Geometry check sheet. Reference: the model listing, model coordinates, mm. Give positions to 0.01 mm unless a question says otherwise; leave off trailing zeros. Write each loop counter-clockwise with the first axis right and the second up, starting at its lowest first coordinate (ties: lowest second). Pieces come first, ordered by that corner, then holes. Notation, with made-up numbers: (71.5, 60.25) - (112.5, 60.25) arc R31 cw to (112.5, 89.25) - close; hole circle Ø4 at (36.25, 39). An arc over 180 degrees is marked (long way). Write item = value, one per line. Start each with the question number.
(1) Section check D-D, the plane y = 29. Enter the section's corners in (x, z), plus the area to 3 significant figures.
(2) Draft check along Y on faces 1 (the cylindrical face through (96, 34, 1)), 2 (the flat face through (109, 50, 2)). Enter one of: pulls with the +Y half, pulls with the -Y half, needs draft (parallel to the pull), parting line crosses it, or undercut.
(3) Depth check by flat-ended pin: pin 1 Ø2.5 at (x, y) = (2.5, 2.5) entering from -Z. Enter the tip coordinate at first touch or a pass-through.
(4) Section check C-C, the plane y = 72. Enter the section's corners in (x, z), plus the area to 3 significant figures.
(5) Thickness scan on L1, parallel to X at y = 95.5, z = 1.4; L2, parallel to Y at x = 2.5, z = 0.65; L3, parallel to Y at x = 94, z = 0.8. Record the ranges inside material, lowest first.
(6) Section check B-B, the plane z = 1.25. Give the number of separate pieces and of enclosed holes in the cut face, plus the area to 3 significant figures.
(7) Section check A-A, the plane x = 60. Enter the section's corners in (y, z), plus the area to 3 significant figures.
```python
from build123d import *

# Parameters (mm, degrees)
SKETCH_1_W      = 180
SKETCH_1_H      = 98
SKETCH_1_R      = 1.5
SKETCH_1_R_2    = 39
SKETCH_1_R_3    = 2
SKETCH_1_R_4    = 1.6
SKETCH_1_W_2    = 27.4
SKETCH_1_H_2    = 47.2
EXTRUDE_1_DEPTH = 2
FILLET_1_R      = 1
FILLET_2_R      = 1


with BuildPart() as part:
    # Эскиз1 → Бобышка-Вытянуть1 (new body)
    with BuildSketch(Plane.XY):
        with Locations((90, 49)):
            Rectangle(SKETCH_1_W, SKETCH_1_H)
        with Locations((2.5, 95.5)):
            Circle(SKETCH_1_R, mode=Mode.SUBTRACT)
        with Locations((177.5, 95.5)):
            Circle(SKETCH_1_R, mode=Mode.SUBTRACT)
        with Locations((177.5, 2.5)):
            Circle(SKETCH_1_R, mode=Mode.SUBTRACT)
        with Locations((2.5, 2.5)):
            Circle(SKETCH_1_R, mode=Mode.SUBTRACT)
        with Locations((60, 49)):
            Circle(SKETCH_1_R_2, mode=Mode.SUBTRACT)
        with Locations((24.25, 84.75)):
            Circle(SKETCH_1_R_3, mode=Mode.SUBTRACT)
        with Locations((95.75, 84.75)):
            Circle(SKETCH_1_R_3, mode=Mode.SUBTRACT)
        with Locations((95.75, 13.25)):
            Circle(SKETCH_1_R_3, mode=Mode.SUBTRACT)
        with Locations((24.25, 13.25)):
            Circle(SKETCH_1_R_3, mode=Mode.SUBTRACT)
        with Locations((125, 64.4)):
            Circle(SKETCH_1_R_4, mode=Mode.SUBTRACT)
        with Locations((165, 64.4)):
            Circle(SKETCH_1_R_4, mode=Mode.SUBTRACT)
        with Locations((145, 64.4)):
            Rectangle(SKETCH_1_W_2, SKETCH_1_H_2, mode=Mode.SUBTRACT)
    extrude(amount=EXTRUDE_1_DEPTH)

    # Скругление1
    fillet_1_edges = [part.edges().sort_by_distance(p)[0] for p in [
        (0, 98, 1),
        (180, 98, 1),
        (180, 0, 1),
        (0, 0, 1),
    ]]
    fillet(fillet_1_edges, radius=FILLET_1_R)

    # Скругление2
    fillet_2_edges = [part.edges().sort_by_distance(p)[0] for p in [
        (158.7, 40.8, 1),
        (158.7, 88, 1),
        (131.3, 88, 1),
        (131.3, 40.8, 1),
    ]]
    fillet(fillet_2_edges, radius=FILLET_2_R)


solid = part.part
```
Model answer:
q1.outline = (0, 0) - (26.52, 0) - (26.52, 2) - (0, 2) - close; (93.48, 0) - (180, 0) - (180, 2) - (93.48, 2) - close
q1.area = 226 mm²
q2.face_1 = undercut
q2.face_2 = needs draft
q3.pin_1 = through
q4.outline = (0, 0) - (28.5, 0) - (28.5, 2) - (0, 2) - close; (91.5, 0) - (131.3, 0) - (131.3, 2) - (91.5, 2) - close; (158.7, 0) - (180, 0) - (180, 2) - (158.7, 2) - close
q4.area = 179 mm²
q5.L1 = 0 to 1, 4 to 176, 179 to 180
q5.L2 = 0 to 1, 4 to 94, 97 to 98
q5.L3 = 0 to 12.28, 14.22 to 29.9, 68.1 to 83.78, 85.72 to 98
q6.separate_pieces = 1
q6.enclosed_holes = 12
q6.area = 11,500 mm²
q7.outline = (0, 0) - (10, 0) - (10, 2) - (0, 2) - close; (88, 0) - (98, 0) - (98, 2) - (88, 2) - close
q7.area = 40.0 mm²
